```python
from build123d import *

# Parameters (mm, degrees)
SKETCH_2_R          = 50
SKETCH_2_R_2        = 30
SKETCH_2_R_3        = 10
EXTRUDE_1_DEPTH     = 10
SKETCH_3_R          = 3
CUT_EXTRUDE_1_DEPTH = 4
SKETCH_4_R          = 1.5
CUT_EXTRUDE_2_DEPTH = 71.964779997
CUT_EXTRUDE_START   = -3
SKETCH_5_R          = 3
CUT_EXTRUDE_3_DEPTH = 3
SKETCH_6_R          = 15
CUT_EXTRUDE_5_DEPTH = 72.414284285


with BuildPart() as part:
    # 草图2 → 凸台-拉伸1 (new body)
    # profile 1 of 2: a face of its own
    with BuildSketch(Plane(origin=(0, 0, 0), x_dir=(1, 0, 0), z_dir=(0, 1, 0))):
        with Locations(Location((0, 0, 0), (0, 0, 270))):
            Circle(SKETCH_2_R)
        Circle(SKETCH_2_R_2, mode=Mode.SUBTRACT)
    # profile 2 of 2: a face of its own
    with BuildSketch(Plane(origin=(0, 0, 0), x_dir=(1, 0, 0), z_dir=(0, 1, 0))):
        Circle(SKETCH_2_R_2)
        with Locations(Location((0, 0, 0), (0, 0, 270))):
            Circle(SKETCH_2_R_3, mode=Mode.SUBTRACT)
    extrude(amount=EXTRUDE_1_DEPTH)

    # 草图3 → 切除-拉伸1 (cut)
    with BuildSketch(Plane(origin=(0, 10, 0), x_dir=(1, 0, 0), z_dir=(0, 1, 0))):
        with Locations(Location((0, 30, 0), (0, 0, 270))):
            Circle(SKETCH_3_R)
        with Locations(Location((30, 0, 0), (0, 0, 270))):
            Circle(SKETCH_3_R)
        with Locations(Location((0, -30, 0), (0, 0, 270))):
            Circle(SKETCH_3_R)
        with Locations(Location((-30, 0, 0), (0, 0, 270))):
            Circle(SKETCH_3_R)
    extrude(amount=-CUT_EXTRUDE_1_DEPTH, mode=Mode.SUBTRACT)

    # 草图4 → 切除-拉伸2 (cut, through all)
    with BuildSketch(Plane(origin=(0, 6, 0), x_dir=(1, 0, 0), z_dir=(0, 1, 0))):
        with Locations(Location((0, 30, 0), (0, 0, 270))):
            Circle(SKETCH_4_R)
        with Locations(Location((30, 0, 0), (0, 0, 270))):
            Circle(SKETCH_4_R)
        with Locations(Location((0, -30, 0), (0, 0, 270))):
            Circle(SKETCH_4_R)
        with Locations(Location((-30, 0, 0), (0, 0, 270))):
            Circle(SKETCH_4_R)
    extrude(amount=-CUT_EXTRUDE_2_DEPTH, mode=Mode.SUBTRACT)

    # 草图5 → 切除-拉伸3 (cut)
    with BuildSketch(Plane.XZ.offset(CUT_EXTRUDE_START)):
        with Locations(Location((0, 30, 0), (0, 0, 90))):
            Circle(SKETCH_5_R)
        with Locations(Location((30, 0, 0), (0, 0, 90))):
            Circle(SKETCH_5_R)
        with Locations(Location((0, -30, 0), (0, 0, 90))):
            Circle(SKETCH_5_R)
        with Locations(Location((-30, 0, 0), (0, 0, 90))):
            Circle(SKETCH_5_R)
    extrude(amount=CUT_EXTRUDE_3_DEPTH, mode=Mode.SUBTRACT)

    # 草图6 → 切除-拉伸5 (cut, through all)
    with BuildSketch(Plane(origin=(0, 10, 0), x_dir=(1, 0, 0), z_dir=(0, 1, 0))):
        with Locations(Location((-21.213203436, 21.213203436, 0), (0, 0, 270))):
            Circle(SKETCH_6_R)
        with BuildLine():
            ThreePointArc((36.213203436, 21.213203436), (35.071396428, 26.953454911), (31.819805169, 31.819805138))
            Line((31.819805153, 31.819805153), (10.606601718, 10.606601718))
            ThreePointArc((10.606601715, 10.606601721), (26.953454919, 7.355010447), (36.213203436, 21.213203436))
        make_face()
        with BuildLine():
            Line((10.606601718, 10.606601718), (31.819805153, 31.819805153))
            ThreePointArc((31.819805169, 31.819805138), (10.606601727, 31.819805163), (10.606601715, 10.606601721))
        make_face()
        with Locations(Location((21.213203436, -21.213203436, 0), (0, 0, 270))):
            Circle(SKETCH_6_R)
        with BuildLine():
            ThreePointArc((-10.60660172, -10.606601716), (-31.819805167, -10.606601732), (-31.819805128, -31.819805179))
            Line((-31.819805153, -31.819805153), (-10.606601718, -10.606601718))
        make_face()
        with BuildLine():
            Line((-10.606601718, -10.606601718), (-31.819805153, -31.819805153))
            ThreePointArc((-31.819805128, -31.819805179), (-15.472951933, -35.071396416), (-6.213203436, -21.213203436))
            ThreePointArc((-6.213203436, -21.213203436), (-7.355010448, -15.472951949), (-10.60660172, -10.606601716))
        make_face()
    extrude(amount=-CUT_EXTRUDE_5_DEPTH, mode=Mode.SUBTRACT)


solid = part.part
```
Work out the finished part from the listing and answer in its coordinate system (mm). A direction names the side the tool comes from. Coordinates: 2 decimals unless noted, no trailing zeros. Write each loop counter-clockwise with the first axis right and the second up, starting at its lowest first coordinate (ties: lowest second). Pieces come first, ordered by that corner, then holes.
Q1. A cutting plane is placed at D-D, the plane x = 5. Give the vertices of the cut face in (y, z).
Q2. Find the intervals of material crossed by line 1 (X direction, y = 1.85, z = 0); line 2 (X direction, y = 2, z = -25); line 3 (Z direction, x = -11, y = 5.5) (3 decimals), in increasing order.
Q3. A cutting plane is placed at A-A, the plane z = 0. State how many separate pieces and enclosed holes the cut face has, then the cut area to 3 significant figures.
Q4. Which of the six approach directions +Z, -Z, +X, -X, +Y, -Y give full straight-line access (tool end or side, diameter ignored) to faces 4 (the face through (0.07, 4.52, 28.5)), 5 (the face through (-29.1, 8.03, 2.86)), 6 (the face through (0, 2, 27))?
Q5. Determine the mould class of faces 1 (the face through (-0.7, 0, 10.4)), 2 (the face through (29.1, 1.52, 2.86)), 3 (the face through (15.02, 4.93, 47.69)) for opening direction Z: released by +Z, released by -Z, zero draft, split by the parting line, or undercut.
Q6. A cutting plane is placed at C-C, the plane x = -14.5. Give the vertices of the cut face in (y, z).
Q7. Each of these flat-tipped pins is pushed along its axis until it touches: pin 1 Ø5 at (y, z) = (5, 1.5) entering from +X; pin 2 Ø1.5 at (x, y) = (10.5, 9) entering from -Z; pin 3 Ø1.8 at (x, z) = (-0.5, -29.5) entering from +Y; pin 4 Ø8 at (x, z) = (0, 30) entering from -Y. Where does it stop, or does it pass through?
Findings below:
1. outline: (0, -49.75) - (10, -49.75) - (10, -8.66) - (0, -8.66) - close; (0, 8.66) - (10, 8.66) - (10, 49.75) - (0, 49.75) - close
2. line 1: x = -50 to -33, -27 to -10, 10 to 27, 33 to 50
2. line 2: x = -43.3 to -35.73, -6.7 to 6.7, 35.73 to 43.3
2. line 3: z = -48.775 to -32.199, -10.227 to 10.227, 32.199 to 48.775
3. separate pieces: 4
3. enclosed holes: 0
3. area: 698 mm2
4. face 4: +Y, -Y
4. face 5: +Y
4. face 6: -Y
5. face 1: zero draft
5. face 2: undercut
5. face 3: split by the parting line
6. outline: (0, -47.85) - (10, -47.85) - (10, -34.63) - (0, -34.63) - close; (0, -7.8) - (10, -7.8) - (10, 7.8) - (0, 7.8) - close; (0, 34.63) - (10, 34.63) - (10, 47.85) - (0, 47.85) - close
7. pin 1: stops at x = 50
7. pin 2: stops at z = -49.04
7. pin 3: stops at y = 6
7. pin 4: stops at y = 0
